CAD build for the part. Positions are in the model's coordinates, mm. A direction names the side the tool comes from. Coordinates: 2 decimals unless noted, no trailing zeros. Loops run counter-clockwise (first coordinate to the right, second up) from the corner with the lowest first, then second, coordinate; pieces in that order, holes last. Notation, with made-up numbers: (-22.5, -21) -> (3.5, -21) arc R23 cw to (3.5, 12) -> close; hole circle Ø3 at (34, 10). An arc over 180 degrees is marked (long way). Write each question's results on one line, items separated by ' | '.
```python
from build123d import *

# Parameters (mm, degrees)
SKETCH1_W              = 150
SKETCH1_H              = 90
BOSS_EXTRUDE1_DEPTH    = 90
SKETCH2_W              = 10
SKETCH2_H              = 40
CUT_EXTRUDE1_DEPTH     = 90
CUT_EXTRUDE2_DEPTH     = 90
CUT_EXTRUDE3_DEPTH     = 10
CUT_EXTRUDE4_DEPTH     = 50
SKETCH6_W              = 10
SKETCH6_H              = 70
CUT_EXTRUDE6_DEPTH     = 94
SKETCH7_R              = 30
CUT_EXTRUDE8_DEPTH     = 10
M20_TAPPED_HOLE2_D     = 17.5
M20_TAPPED_HOLE2_DEPTH = 25
M20_TAPPED_HOLE2_TIP   = 5.257530416
M20_TAPPED_HOLE3_D     = 17.5
M20_TAPPED_HOLE3_DEPTH = 37.5
M20_TAPPED_HOLE3_TIP   = 5.257530416


with BuildPart() as part:
    # Sketch1 → Boss-Extrude1 (new body)
    with BuildSketch(Plane.XY):
        with Locations((75, 45)):
            Rectangle(SKETCH1_W, SKETCH1_H)
    extrude(amount=BOSS_EXTRUDE1_DEPTH)

    # Sketch2 → Cut-Extrude1 (cut)
    with BuildSketch(Plane.XY.offset(90)):
        with Locations((145, 45)):
            Rectangle(SKETCH2_W, SKETCH2_H)
    extrude(amount=-CUT_EXTRUDE1_DEPTH, mode=Mode.SUBTRACT)

    # Sketch3 → Cut-Extrude2 (cut)
    with BuildSketch(Plane.XY.offset(90)):
        with BuildLine():
            ThreePointArc((0, 45), (13.180194847, 76.819805153), (45, 90))
            Line((45, 90), (0, 90))
            Line((0, 90), (0, 45))
        make_face()
        with BuildLine():
            ThreePointArc((45, 0), (13.180194847, 13.180194847), (0, 45))
            Line((0, 45), (0, 0))
            Line((0, 0), (45, 0))
        make_face()
    extrude(amount=-CUT_EXTRUDE2_DEPTH, mode=Mode.SUBTRACT)

    # Sketch4 → Cut-Extrude3 (cut)
    with BuildSketch(Plane(origin=(0, 0, 0), x_dir=(-1, 0, 0), z_dir=(0, 0, -1))):
        with BuildLine():
            ThreePointArc((-11.458980338, 15), (0, 45), (-11.458980338, 75))
            Line((-11.458980338, 75), (-45, 75))
            ThreePointArc((-45, 75), (-75, 45), (-45, 15))
            Line((-45, 15), (-11.458980338, 15))
        make_face()
    extrude(amount=-CUT_EXTRUDE3_DEPTH, mode=Mode.SUBTRACT)

    # Sketch5 → Cut-Extrude4 (cut)
    with BuildSketch(Plane.XY.offset(90)):
        with BuildLine():
            Line((95, 90), (95, 0))
            Line((95, 0), (45, 0))
            ThreePointArc((45, 0), (0, 45), (45, 90))
            Line((45, 90), (95, 90))
        make_face()
    extrude(amount=-CUT_EXTRUDE4_DEPTH, mode=Mode.SUBTRACT)

    # Sketch6 → Cut-Extrude6 (cut)
    with BuildSketch(Plane.ZY.offset(-95)):
        with Locations((85, 45)):
            Rectangle(SKETCH6_W, SKETCH6_H)
    extrude(amount=-CUT_EXTRUDE6_DEPTH, mode=Mode.SUBTRACT)

    # Sketch7 → Cut-Extrude8 (cut)
    with BuildSketch(Plane.XY.offset(40)):
        with Locations((45, 45)):
            Circle(SKETCH7_R)
        with BuildLine():
            Line((95, 65), (67.360679775, 65))
            ThreePointArc((67.360679775, 65), (73.025170769, 55.704662693), (75, 45))
            ThreePointArc((75, 45), (73.025170769, 34.295337307), (67.360679775, 25))
            Line((67.360679775, 25), (95, 25))
            Line((95, 25), (95, 65))
        make_face()
    extrude(amount=-CUT_EXTRUDE8_DEPTH, mode=Mode.SUBTRACT)

    # M20 Tapped Hole2
    with Locations(Plane(origin=(115, 65, 80), x_dir=(0, 1, 0), z_dir=(0, 0, 1))):
        with Locations((0, 0), (-40, 0)):
            Hole(M20_TAPPED_HOLE2_D / 2, depth=M20_TAPPED_HOLE2_DEPTH)
            with Locations((0, 0, -(M20_TAPPED_HOLE2_DEPTH + M20_TAPPED_HOLE2_TIP / 2))):  # 118° drill point
                Cone(0, M20_TAPPED_HOLE2_D / 2, M20_TAPPED_HOLE2_TIP, mode=Mode.SUBTRACT)

    # M20 Tapped Hole3
    with Locations(Plane(origin=(45, 45, 40), x_dir=(1, 0, 0), z_dir=(0, 0, 1))):
        with Locations((0, 0)):
            Hole(M20_TAPPED_HOLE3_D / 2, depth=M20_TAPPED_HOLE3_DEPTH)
            with Locations((0, 0, -(M20_TAPPED_HOLE3_DEPTH + M20_TAPPED_HOLE3_TIP / 2))):  # 118° drill point
                Cone(0, M20_TAPPED_HOLE3_D / 2, M20_TAPPED_HOLE3_TIP, mode=Mode.SUBTRACT)


solid = part.part
```
Q1. Cut at C-C on y = 48. Write the cut outline in (x, z).
Results are:
outline: (0.1, 10) -> (36.78, 10) -> (36.78, 30) -> (15.15, 30) -> (15.15, 40) -> (0.1, 40) -> close; (53.22, 10) -> (74.85, 10) -> (74.85, 0) -> (140, 0) -> (140, 80) -> (95, 80) -> (95, 30) -> (53.22, 30) -> close
Q2. Which spindle directions (+Z, -Z, +X, -X, +Y, -Y) get a long thin tool onto all of the face, cutting with end or side? Do faces 1 (the flat face through (48, 76, 40)), 2 (the flat face through (122, 85, 90)), 3 (the flat face through (54, 45, 30)), 4 (the flat face through (122, 10, 85)), 5 (the flat face through (28, 15, 5)). Say none if no direction does.
Results are:
face 1: +Z, -X, +Y, -Y | face 2: +Z, +X, -X, +Y, -Y | face 3: +Z | face 4: +Z, +X, -X | face 5: -Z, -X
Q3. Cut at A-A on z = 84. Write the cut outline in (x, y), and give its area (3 significant figures).
Results are:
outline: (95, 0) -> (150, 0) -> (150, 10) -> (95, 10) -> close; (95, 80) -> (150, 80) -> (150, 90) -> (95, 90) -> close | area: 1,100 mm^2
Q4. Cut at D-D on x = 73. Write the cut outline in (y, z), and give its area (3 significant figures).
Results are:
outline: (0, 0) -> (34.23, 0) -> (34.23, 10) -> (55.77, 10) -> (55.77, 0) -> (90, 0) -> (90, 40) -> (65, 40) -> (65, 30) -> (25, 30) -> (25, 40) -> (0, 40) -> close | area: 2,980 mm^2
Q5. Pull direction Y, two halves, no side cores. Call faces 6 (the flat face through (145, 25, 41)), 7 (the flat face through (122, 5, 90)): +Y half, -Y half, draft (parallel to the pull), parting line (faces both ways), or undercut.
Results are:
face 6: undercut | face 7: draft
Q6. Drop flat-ended pins along their axis: pin 1 (5 mm diameter, centred on x = 18, z = 36, fed in from -Y); pin 2 (16 mm diameter, centred on x = 115, y = 65, fed in from +Z); pin 3 (6 mm diameter, centred on x = 21, z = 36.5, fed in from -Y). Give the stop position or say it passes through.
Results are:
pin 1: y = 7.25 | pin 2: z = 54.55 | pin 3: y = 5.2
Q7. Cut at B-B on z = 60.5. Write the cut outline in (x, y), and give its area (3 significant figures).
Results are:
outline: (95, 0) -> (150, 0) -> (150, 25) -> (140, 25) -> (140, 65) -> (150, 65) -> (150, 90) -> (95, 90) -> close; hole circle Ø17.5 at (115, 25); hole circle Ø17.5 at (115, 65) | area: 4,070 mm^2
Q8. Wall check: L1, parallel to Y at x = 115, z = 70.25; L2, parallel to X at y = 45, z = 32.25; L3, parallel to Y at x = 45, z = 35. Give the ranges that are in metal, low to high. Write a range as from..to.
Results are:
L1: 0..16.25, 33.75..56.25, 73.75..90 | L2: 0..15, 95..140 | L3: 0..15, 75..90
